Check sheet for the drawn part. Datum: minimum x, y, z corner. Units: mm. Round coordinates to 2 decimals unless told otherwise and drop trailing zeros. Write each loop counter-clockwise with the first axis right and the second up, starting at its lowest first coordinate (ties: lowest second). Pieces come first, ordered by that corner, then holes.
Item 1: Material ranges on line 1 (Z direction, x = 256, y = 303), recorded low to high.
Item 2: Cross-section at B-B on x = 223. Enter the section's corners in (y, z), plus the area to 3 significant figures.
Item 3: Go/stop test with a flat-tipped pin: pin 1 Ø5 at (x, y) = (102, 338) entering from -Z. Record where the tip stops, or that it passes through.
Item 4: Cross-section at C-C on y = 68.5. Enter the section's corners in (x, z), plus the area to 3 significant figures.
Item 5: Cross-section at A-A on z = 147. Enter the section's corners in (x, y), plus the area to 3 significant figures.
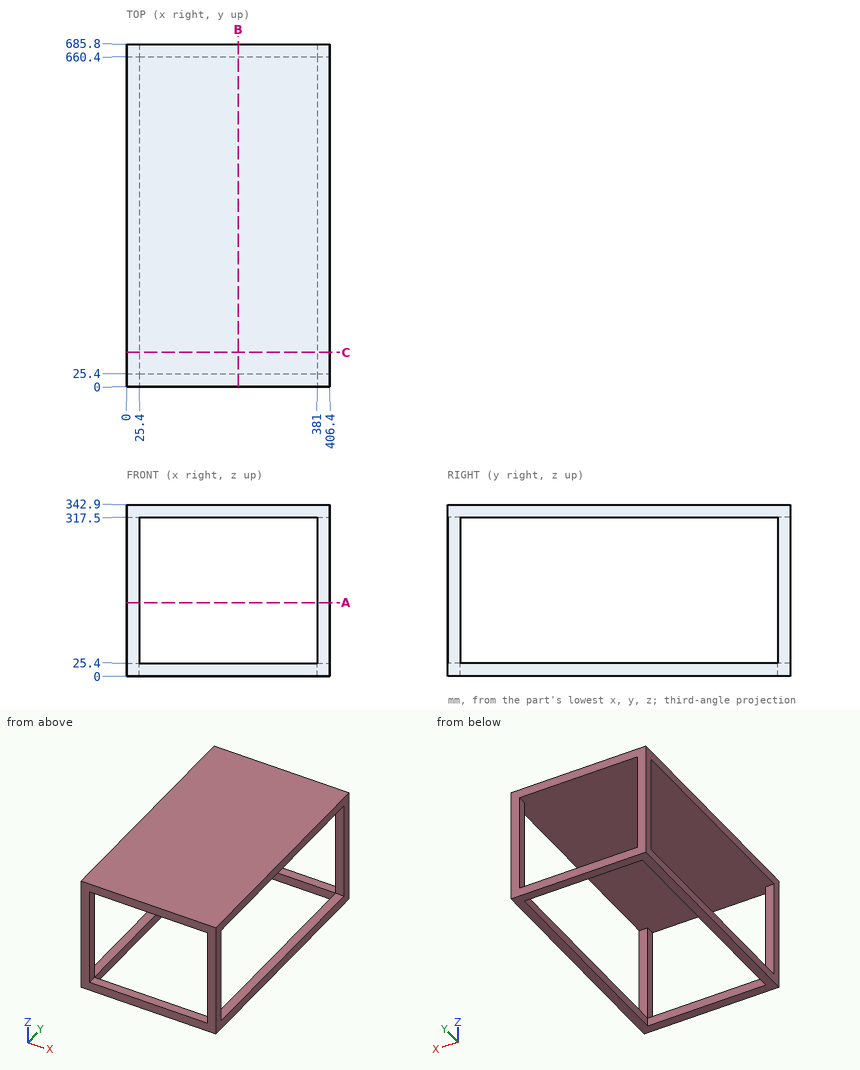
Response values:
1. line 1: z = 317.5 to 342.9
2. outline: (0, 0) - (25.4, 0) - (25.4, 25.4) - (0, 25.4) - close; (0, 317.5) - (685.8, 317.5) - (685.8, 342.9) - (0, 342.9) - close; (660.4, 0) - (685.8, 0) - (685.8, 25.4) - (660.4, 25.4) - close
2. area: 18,700 mm2
3. pin 1: stops at z = 317.5
4. outline: (0, 0) - (25.4, 0) - (25.4, 25.4) - (0, 25.4) - close; (0, 317.5) - (406.4, 317.5) - (406.4, 342.9) - (0, 342.9) - close; (381, 0) - (406.4, 0) - (406.4, 25.4) - (381, 25.4) - close
4. area: 11,600 mm2
5. outline: (0, 0) - (25.4, 0) - (25.4, 25.4) - (0, 25.4) - close; (0, 660.4) - (25.4, 660.4) - (25.4, 685.8) - (0, 685.8) - close; (381, 0) - (406.4, 0) - (406.4, 25.4) - (381, 25.4) - close; (381, 660.4) - (406.4, 660.4) - (406.4, 685.8) - (381, 685.8) - close
5. area: 2,580 mm2
